from build123d import *

# Parameters (mm, degrees)
SKETCH1_W               = 40
SKETCH1_H               = 36
SKETCH1_W_2             = 32
SKETCH1_H_2             = 28.8
BOSS_EXTRUDE1_DEPTH     = 530
SKETCH2_W               = 50
SKETCH2_H               = 28.8
CUT_EXTRUDE1_DEPTH      = 40
FILLET2_RADIUS          = 20
FILLET2_LENGTH          = 3.6
FILLET3_RADIUS          = 20
FILLET3_LENGTH          = 3.6
CUT_EXTRUDE2_DEPTH      = 532.597592169
CUT_EXTRUDE2_DEPTH_BACK = 532.597592169
SKETCH3_R               = 6
CUT_EXTRUDE3_DEPTH      = 10
SKETCH12_R              = 2.5
BOSS_EXTRUDE3_DEPTH     = 36
CUT_EXTRUDE6_START      = -9
SKETCH13_R              = 5
CUT_EXTRUDE6_DEPTH      = 9
CUT_EXTRUDE7_START      = -9
SKETCH14_R              = 5
CUT_EXTRUDE7_DEPTH      = 9
FILLET6_R               = 1


with BuildPart() as part:
    # Sketch1 → Boss-Extrude1 (new body)
    with BuildSketch(Plane.XY):
        Rectangle(SKETCH1_W, SKETCH1_H)
        Rectangle(SKETCH1_W_2, SKETCH1_H_2, mode=Mode.SUBTRACT)
    extrude(amount=BOSS_EXTRUDE1_DEPTH)

    # Sketch2 → Cut-Extrude1 (cut)
    with BuildSketch(Plane.XY.offset(530)):
        Rectangle(SKETCH2_W, SKETCH2_H)
    extrude(amount=-CUT_EXTRUDE1_DEPTH, mode=Mode.SUBTRACT)

    # Fillet2: full round fillet: the end face becomes a half cylinder, R = half its width
    fillet2_face = Plane((0, -16.2, 530), x_dir=(0, -1, 0), z_dir=(0, 0, 1))  # on the end face: x along it, z out of the body
    fillet2_slab = fillet2_face.offset(-FILLET2_RADIUS / 2) * Box(FILLET2_LENGTH, 2 * FILLET2_RADIUS, FILLET2_RADIUS, mode=Mode.PRIVATE)  # the body's end, R deep
    fillet2_round = Plane((0, -16.2, 510), x_dir=(0, 0, 1), z_dir=(0, -1, 0)) * Cylinder(FILLET2_RADIUS, FILLET2_LENGTH, mode=Mode.PRIVATE)  # its axis R under the face
    add(fillet2_slab - fillet2_round, mode=Mode.SUBTRACT)

    # Fillet3: full round fillet: the end face becomes a half cylinder, R = half its width
    fillet3_face = Plane((0, 16.2, 530), x_dir=(0, -1, 0), z_dir=(0, 0, 1))  # on the end face: x along it, z out of the body
    fillet3_slab = fillet3_face.offset(-FILLET3_RADIUS / 2) * Box(FILLET3_LENGTH, 2 * FILLET3_RADIUS, FILLET3_RADIUS, mode=Mode.PRIVATE)  # the body's end, R deep
    fillet3_round = Plane((0, 16.2, 510), x_dir=(0, 0, 1), z_dir=(0, -1, 0)) * Cylinder(FILLET3_RADIUS, FILLET3_LENGTH, mode=Mode.PRIVATE)  # its axis R under the face
    add(fillet3_slab - fillet3_round, mode=Mode.SUBTRACT)

    # Sketch3 → Cut-Extrude2 (cut, two sides: drawn at the far end of the back side and taken through both)
    with BuildSketch(Plane(origin=(0, 18, 0), x_dir=(1, 0, 0), z_dir=(0, 1, 0)).offset(-CUT_EXTRUDE2_DEPTH_BACK)):
        with Locations(Location((0, -510, 0), (0, 0, 270))):
            Circle(SKETCH3_R)
    extrude(amount=CUT_EXTRUDE2_DEPTH + CUT_EXTRUDE2_DEPTH_BACK, mode=Mode.SUBTRACT)

    # Sketch6 → Cut-Extrude3 (cut)
    with BuildSketch(Plane.XZ.offset(18)):
        with BuildLine():
            ThreePointArc((6, 460), (0, 466), (-6, 460))
            Line((-6, 460), (-6, 360))
            ThreePointArc((-6, 360), (0, 354), (6, 360))
            Line((6, 360), (6, 460))
        make_face()
    extrude(amount=-CUT_EXTRUDE3_DEPTH, mode=Mode.SUBTRACT)

    # Sketch12 → Boss-Extrude3 (add)
    with BuildSketch(Plane.XZ.offset(18)):
        with BuildLine():
            Line((-20, 0), (-20, 40))
            Line((-20, 40), (-22.5, 40))
            Line((-22.5, 40), (-22.5, 4.330127019))
            ThreePointArc((-22.5, 4.330127019), (-29.330127019, -2.5), (-20, 0))
        make_face()
        with Locations(Location((-25, 0, 0), (0, 0, 270))):
            Circle(SKETCH12_R, mode=Mode.SUBTRACT)
    extrude(amount=-BOSS_EXTRUDE3_DEPTH)

    # Sketch13 → Cut-Extrude6 (cut)
    with BuildSketch(Plane(origin=(0, 18, 0), x_dir=(1, 0, 0), z_dir=(0, 1, 0)).offset(CUT_EXTRUDE6_START)):
        with Locations((-25, 0)):
            Circle(SKETCH13_R)
    extrude(amount=CUT_EXTRUDE6_DEPTH, mode=Mode.SUBTRACT)

    # Sketch14 → Cut-Extrude7 (cut)
    with BuildSketch(Plane(origin=(0, 0, 0), x_dir=(1, 0, 0), z_dir=(0, 1, 0)).offset(CUT_EXTRUDE7_START)):
        with Locations((-25, 0)):
            Circle(SKETCH14_R)
    extrude(amount=CUT_EXTRUDE7_DEPTH, mode=Mode.SUBTRACT)

    # Fillet6
    fillet6_edges = [part.edges().sort_by_distance(p)[0] for p in [
        (-22.5, 0, 40),
    ]]
    fillet(fillet6_edges, radius=FILLET6_R)


solid = part.part
Read the model definition and answer for the solid it produces. Units are mm, in the model's axes. A direction names the side the tool comes from. Round coordinates to 2 decimals unless told otherwise and drop trailing zeros. Order: outer loops, then holes, each group sorted by start corner. A loop starts at its lowest first (then second) coordinate and runs counter-clockwise, first axis right, second up. Notation, with made-up numbers: (73, 71) - (82, 71) arc R21 cw to (82, 99) - close; hole circle Ø5 at (26.25, -30). An arc over 180 degrees is marked (long way). Use one line per item in the form item = value. Start each with the question number.
(1) The part is cut by section B-B (z = 276.5). Give the vertices of the cut face in (x, y), then the cut area to 3 significant figures.
(2) Flat-ended cylindrical pins translate along their axes: pin 1 Ø14.5 at (y, z) = (-0.5, 296) entering from -X; pin 2 Ø3 at (x, z) = (-26, -2) entering from +Y; pin 3 Ø6 at (x, y) = (2.5, -14) entering from +Z. Find the tip coordinate at first contact, or state that the pin passes through.
(3) Determine the mould class of faces 5 (the face through (0, -18, 266)), 6 (the face through (0, -14.4, 269)), 7 (the face through (0, -16, 504)), 8 (the face through (-23, -9, 2)) for opening direction Y: +Y half, -Y half, draft (parallel to the pull), parting line (faces both ways), or undercut.
(4) The part is cut by section A-A (x = 0). Give the vertices of the cut face in (y, z).
(5) Find the intervals of material crossed by line 1 along Z through (x, y) = (0, 15); line 2 along X through (y, z) = (-8, 209); line 3 along Y through (x, z) = (-4, 328.5), in increasing order. Write a range as from..to.
(6) The part is cut by section C-C (z = 425). Give the vertices of the cut face in (x, y), then the cut area to 3 significant figures.
(7) For faces 1 (the face through (-23, 9, 2)), 2 (the face through (0, -16, 0)), 3 (the face through (-23, 0, 2)), 4 (the face through (16, 0, 242)), determine the directions among +Z, -Z, +X, -X, +Y, -Y from which every point of the face is accessible in a straight line to the end or side of a thin tool.
Checked values:
q1.outline = (-20, -18) - (20, -18) - (20, 18) - (-20, 18) - close; hole (-16, -14.4) - (16, -14.4) - (16, 14.4) - (-16, 14.4) - close
q1.area = 518 mm^2
q2.pin_1 = -20
q2.pin_2 = 9
q2.pin_3 = 530
q3.face_5 = -Y half
q3.face_6 = undercut
q3.face_7 = draft
q3.face_8 = undercut
q4.outline = (-18, 0) - (-14.4, 0) - (-14.4, 354) - (-18, 354) - close; (-18, 466) - (-14.4, 466) - (-14.4, 504) - (-18, 504) - close; (-18, 516) - (-14.4, 516) - (-14.4, 530) - (-18, 530) - close; (14.4, 0) - (18, 0) - (18, 504) - (14.4, 504) - close; (14.4, 516) - (18, 516) - (18, 530) - (14.4, 530) - close
q5.line_1 = 0..504, 516..530
q5.line_2 = -20..-16, 16..20
q5.line_3 = -18..-14.4, 14.4..18
q6.outline = (-20, -18) - (-6, -18) - (-6, -14.4) - (-16, -14.4) - (-16, 14.4) - (16, 14.4) - (16, -14.4) - (6, -14.4) - (6, -18) - (20, -18) - (20, 18) - (-20, 18) - close
q6.area = 475 mm^2
q7.face_1 = -Z, -X, +Y
q7.face_2 = -Z, +X, +Y, -Y
q7.face_3 = -Z, -X
q7.face_4 = +Z, -Z
